Input: part model. Units: mm. Frame: model coordinates. Face numbers are marked on the shaded views. Coordinates: 2 decimals unless noted, no trailing zeros. Write each loop counter-clockwise with the first axis right and the second up, starting at its lowest first coordinate (ties: lowest second). Pieces come first, ordered by that corner, then holes. Notation, with made-up numbers: M -32.5,-8 L 5.5,-8 A21 cw 5.5,6 Z; hole C -10.75,27 d2. An arc over 180 degrees is marked long. Answer as a JSON object with one key per item and string values. Group by question number.
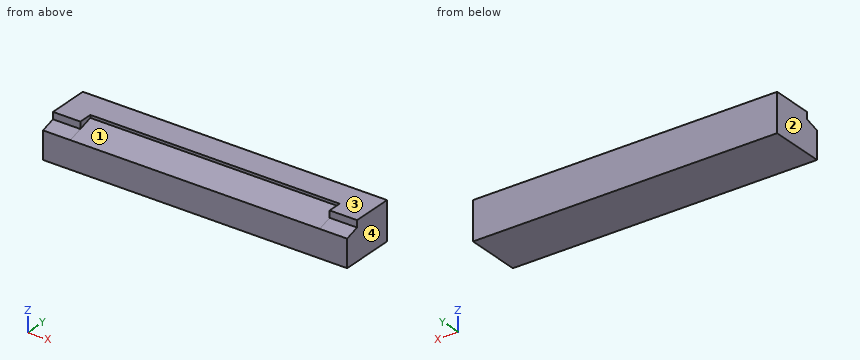
from build123d import *

# Parameters (mm, degrees)
F1_DEPTH = 455
F3_DEPTH = 100


with BuildPart() as f1:
    # F0 (on Right) → F1 (new body)
    with BuildSketch(Plane.YZ):
        Polygon((100, 31.431883), (0, 31.431883), (0, 21.431883), (-99.810627, -8.568117), (-99.810627, -108.568117), (100, -108.568117), align=None)
    extrude(amount=F1_DEPTH)

    # F2 (on face) → F3 (join)
    with BuildSketch(Plane.YZ.offset(455)):
        Polygon((-99.810627, -108.568117), (100, -108.568117), (100, 31.431883), (0, 31.431883), (0, 21.431883), (-50, 6.403424), (-99.810627, -8.568117), align=None)
        Polygon((0, 21.431883), (0, 31.431883), (-50, 31.431883), (-50, 6.403424), align=None)
    extrude(amount=F3_DEPTH)

    # F4: F1 across face


with BuildPart() as f1_1:
    add(f1.part)
    add(f1.part.mirror(Plane(origin=(0, 5.969064, -44.0526), x_dir=(0, 1, 0), z_dir=(-1, 0, 0))))


solid = f1_1.part
Q1. Line query: line 1 (X direction, y = -48.5, z = 14.5); line 2 (Y direction, x = -32, z = 21.5); line 3 (Z direction, x = 440.5, y = -90.5). Output: solid intervals per line, ascending. Write a range as from..to.
Q2. Draft query along X for the marked faces 1, 2, 3 and 4. Return one class per face: released by +X, released by -X, zero draft, split by the parting line, or undercut.
Q3. Section C-C, the plane y = -77. Return the cut outline in (x, z).
Q4. Section B-B, the plane y = -24.5. Return the cut outline in (x, z), and give its area (3 significant figures).
Q5. Pin query (flat end, axial travel): pin 1 Ø5 at (x, z) = (-175, 25.5) entering from -Y; pin 2 Ø4 at (x, y) = (178.5, -53.5) entering from +Z; pin 3 Ø20 at (x, z) = (497, 17) entering from -Y. Return the tip coordinate at first contact, or that it passes through.
Q6. Section A-A, the plane x = 75. Return the cut outline in (y, z).
Filled in:
{
 "1": {"line 1": "-555..-455, 455..555", "line 2": "0..100", "line 3": "-108.57..-5.77"},
 "2": {"face 1": "undercut", "face 2": "released by -X", "face 3": "zero draft", "face 4": "released by +X"},
 "3": {"outline": "M -555,-108.57 L 555,-108.57 L 555,-1.71 L -555,-1.71 Z"},
 "4": {"outline": "M -555,-108.57 L 555,-108.57 L 555,31.43 L 455,31.43 L 455,14.07 L -455,14.07 L -455,31.43 L -555,31.43 Z", "area": "140,000 mm^2"},
 "5": {"pin 1": "y = 0", "pin 2": "z = 5.95", "pin 3": "y = -50"},
 "6": {"outline": "M -99.81,-108.57 L 100,-108.57 L 100,31.43 L 0,31.43 L 0,21.43 L -99.81,-8.57 Z"}
}
